Model file for the job. Use its own axes, mm. A direction names the side the tool comes from. Give positions to 0.01 mm unless a question says otherwise; leave off trailing zeros. Loops run counter-clockwise (first coordinate to the right, second up) from the corner with the lowest first, then second, coordinate; pieces in that order, holes last. Notation, with made-up numbers: M -37,33.5 L -25,33.5 A22 ccw -25,68.5 Z; hole C 4,22 d9. An arc over 180 degrees is marked long. Answer in a Markdown table with one row per item.
```python
from build123d import *

# Parameters (mm, degrees)
SKETCH3_W               = 50
SKETCH3_H               = 50
BOSS_EXTRUDE1_DEPTH     = 5
BOSS_EXTRUDE4_START     = 5
SKETCH4_W               = 30
SKETCH4_H               = 33.5
BOSS_EXTRUDE4_DEPTH     = 70
CUT_EXTRUDE1_START      = 2
SKETCH6_W               = 20
SKETCH6_H               = 41
CUT_EXTRUDE1_DEPTH      = 19
SKETCH7_W               = 30
SKETCH7_H               = 15
CUT_EXTRUDE2_DEPTH      = 26
CUT_EXTRUDE2_DEPTH_BACK = 26
SKETCH9_R               = 1.55
CUT_EXTRUDE4_DEPTH      = 26
CUT_EXTRUDE4_DEPTH_BACK = 26
SKETCH10_R              = 1.55
CUT_EXTRUDE6_DEPTH      = 61
CUT_EXTRUDE6_DEPTH_BACK = 1
SKETCH11_W              = 50
SKETCH11_H              = 8.193147868
CUT_EXTRUDE7_DEPTH      = 25
SKETCH12_R              = 1.55
CUT_EXTRUDE8_DEPTH      = 61
CUT_EXTRUDE8_DEPTH_BACK = 25


with BuildPart() as part:
    # Sketch3 → Boss-Extrude1 (new body)
    with BuildSketch(Plane.XY):
        Rectangle(SKETCH3_W, SKETCH3_H)
    extrude(amount=BOSS_EXTRUDE1_DEPTH)

    # Sketch4 → Boss-Extrude4 (add)
    with BuildSketch(Plane.XY.offset(BOSS_EXTRUDE4_START)):
        Rectangle(SKETCH4_W, SKETCH4_H)
    extrude(amount=BOSS_EXTRUDE4_DEPTH)

    # Sketch6 → Cut-Extrude1 (cut)
    with BuildSketch(Plane(origin=(0, 0, 0), x_dir=(1, 0, 0), z_dir=(0, 1, 0)).offset(CUT_EXTRUDE1_START)):
        with Locations((0, -35.5)):
            Rectangle(SKETCH6_W, SKETCH6_H)
    extrude(amount=-CUT_EXTRUDE1_DEPTH, mode=Mode.SUBTRACT)

    # Sketch7 → Cut-Extrude2 (cut, two sides)
    with BuildSketch(Plane(origin=(0, 0, 0), x_dir=(1, 0, 0), z_dir=(0, 1, 0))) as cut_extrude2_sk:
        with Locations((0, -67.5)):
            Rectangle(SKETCH7_W, SKETCH7_H)
    extrude(amount=CUT_EXTRUDE2_DEPTH, mode=Mode.SUBTRACT)
    extrude(cut_extrude2_sk.sketch, amount=-CUT_EXTRUDE2_DEPTH_BACK, mode=Mode.SUBTRACT)

    # Sketch9 → Cut-Extrude4 (cut, two sides)
    with BuildSketch(Plane(origin=(0, 0, 0), x_dir=(0, 0, -1), z_dir=(1, 0, 0))) as cut_extrude4_sk:
        with Locations((-25, 11.75)):
            Circle(SKETCH9_R)
        with Locations((-15, 11.75)):
            Circle(SKETCH9_R)
    extrude(amount=CUT_EXTRUDE4_DEPTH, mode=Mode.SUBTRACT)
    extrude(cut_extrude4_sk.sketch, amount=-CUT_EXTRUDE4_DEPTH_BACK, mode=Mode.SUBTRACT)

    # Sketch10 → Cut-Extrude6 (cut, two sides)
    with BuildSketch(Plane.XY) as cut_extrude6_sk:
        with BuildLine():
            Line((-20.096015511, 20.096015511), (-17.903984489, 17.903984489))
            ThreePointArc((-17.903984489, 17.903984489), (-17.903984489, 20.096015511), (-20.096015511, 20.096015511))
        make_face()
        with Locations((19, 19)):
            Circle(SKETCH10_R)
        with Locations((19, -19)):
            Circle(SKETCH10_R)
        with Locations((-19, -19)):
            Circle(SKETCH10_R)
    extrude(amount=CUT_EXTRUDE6_DEPTH, mode=Mode.SUBTRACT)
    extrude(cut_extrude6_sk.sketch, amount=-CUT_EXTRUDE6_DEPTH_BACK, mode=Mode.SUBTRACT)

    # Sketch11 → Cut-Extrude7 (cut)
    with BuildSketch(Plane.XY.offset(5)):
        with Locations((0, 20.903426066)):
            Rectangle(SKETCH11_W, SKETCH11_H)
    extrude(amount=-CUT_EXTRUDE7_DEPTH, mode=Mode.SUBTRACT)

    # Sketch12 → Cut-Extrude8 (cut, two sides)
    with BuildSketch(Plane.XY) as cut_extrude8_sk:
        with Locations((-19, 11.806852132)):
            Circle(SKETCH12_R)
        with Locations((19, 11.806852132)):
            Circle(SKETCH12_R)
    extrude(amount=CUT_EXTRUDE8_DEPTH, mode=Mode.SUBTRACT)
    extrude(cut_extrude8_sk.sketch, amount=-CUT_EXTRUDE8_DEPTH_BACK, mode=Mode.SUBTRACT)


solid = part.part
```
(1) Saw through at A-A, the plane x = -19. Give the cut face in (y, z).
Established:
| item | result |
|---|---|
| outline | M -25,0 L -20.55,0 L -20.55,5 L -25,5 Z; M -17.45,0 L 10.26,0 L 10.26,5 L -17.45,5 Z; M 13.36,0 L 16.81,0 L 16.81,5 L 13.36,5 Z |
(2) Which spindle directions (+Z, -Z, +X, -X, +Y, -Y) get a long thin tool onto all of the face, cutting with end or side? Do faces 5 (the flat face through (0, -7, 15)), 6 (the flat face through (-10.2, -16.75, 32.1)), 7 (the flat face through (0, 16.75, 32)), 8 (the flat face through (15, 0, 32)), 9 (the flat face through (-15, 0, 32)). Say none if no direction does.
Established:
| item | result |
|---|---|
| face 5 | -Y |
| face 6 | +Z, +X, -X, -Y |
| face 7 | +Z, +X, -X, +Y |
| face 8 | +Z, +X, +Y, -Y |
| face 9 | +Z, -X, +Y, -Y |
(3) Saw through at D-D, the plane y = -19. Give the cut face in (x, z), and give its area (3 significant figures).
Established:
| item | result |
|---|---|
| outline | M -25,0 L -20.55,0 L -20.55,5 L -25,5 Z; M -17.45,0 L 17.45,0 L 17.45,5 L -17.45,5 Z; M 20.55,0 L 25,0 L 25,5 L 20.55,5 Z |
| area | 219 mm2 |
(4) Saw through at B-B, the plane z = 25. Give the cut face in (x, y).
Established:
| item | result |
|---|---|
| outline | M -15,-16.75 L -10,-16.75 L -10,2 L 10,2 L 10,-16.75 L 15,-16.75 L 15,10.2 L -15,10.2 Z; M -15,13.3 L 15,13.3 L 15,16.75 L -15,16.75 Z |
(5) Flat gauge pins, fed straight in: P1, Ø4, axis at y = -12.5, z = 32, coming from the -X side; P2, Ø2, axis at x = 17.5, y = 6, coming from the -Z side; P3, Ø1, axis at x = 2, z = 46, coming from the +Y side; P4, Ø5.5, axis at y = -3, z = 34, coming from the +X side. Where does each tip first touch, or does it go through?
Established:
| item | result |
|---|---|
| P1 | stops at x = -15 |
| P2 | stops at z = 0 |
| P3 | stops at y = 16.75 |
| P4 | stops at x = 15 |
(6) Wall check: L1, parallel to Z at x = -1.25, y = 11.75; L2, parallel to Y at x = 19, z = 2.8; L3, parallel to Z at x = 0.5, y = -5. Give the ranges that are in metal, low to high.
Established:
| item | result |
|---|---|
| L1 | z = 0 to 13.45, 16.55 to 23.45, 26.55 to 60 |
| L2 | y = -25 to -20.55, -17.45 to 10.26, 13.36 to 16.81 |
| L3 | z = 0 to 15, 56 to 60 |
(7) Mould opens along Y. For faces 1 (the cylindrical face through (0.21, 11.82, 16.55)), 2 (the cylindrical face through (0.21, 10.237, 25.336)), 3 (the flat face through (0, 2, 35)), 4 (the flat face through (10, -7, 36)) say: pulls with the +Y half, pulls with the -Y half, needs draft (parallel to the pull), parting line crosses it, or undercut.
Established:
| item | result |
|---|---|
| face 1 | undercut |
| face 2 | undercut |
| face 3 | pulls with the -Y half |
| face 4 | needs draft |
(8) Saw through at C-C, the plane x = -8.5. Give the cut face in (y, z), and give its area (3 significant figures).
Established:
| item | result |
|---|---|
| outline | M -25,0 L 16.81,0 L 16.81,5 L 16.75,5 L 16.75,60 L -16.75,60 L -16.75,56 L 2,56 L 2,15 L -16.75,15 L -16.75,5 L -25,5 Z; hole C 11.75,15 d3.1; hole C 11.75,25 d3.1 |
| area | 1,270 mm2 |
